CAD build for the part. Positions are in the model's coordinates, mm. Face numbers are marked on the shaded views. A direction names the side the tool comes from. Coordinates: 2 decimals unless noted, no trailing zeros. Loops run counter-clockwise (first coordinate to the right, second up) from the corner with the lowest first, then second, coordinate; pieces in that order, holes last. Notation, with made-up numbers: (86.25, 16) -> (118.25, 16) arc R21 ccw to (118.25, 29) -> close; hole circle Ø2 at (59, 41). An arc over 180 degrees is marked (long way). Write each question's results on one line, items separated by ' | '.
from build123d import *

# Parameters (mm, degrees)
SKETCH1_W           = 8
SKETCH1_H           = 40
BOSS_EXTRUDE1_DEPTH = 5
SKETCH3_W           = 8
SKETCH3_H           = 8
BOSS_EXTRUDE3_DEPTH = 70
SKETCH4_R           = 4
BOSS_EXTRUDE4_DEPTH = 30
SKETCH5_R           = 0.773565548
SKETCH5_R_2         = 0.768304054
SKETCH5_R_3         = 0.726526648
SKETCH5_R_4         = 0.707209462
SKETCH5_R_5         = 0.715862797
SKETCH5_R_6         = 0.812614346
CUT_EXTRUDE1_DEPTH  = 10
FILLET1_R           = 3


with BuildPart() as part:
    # Sketch1 → Boss-Extrude1 (new body)
    with BuildSketch(Plane.XY):
        with Locations((4, 20)):
            Rectangle(SKETCH1_W, SKETCH1_H)
    extrude(amount=BOSS_EXTRUDE1_DEPTH)

    # Sketch3 → Boss-Extrude3 (add)
    with BuildSketch(Plane.XY.offset(5)):
        with Locations((4, 20)):
            Rectangle(SKETCH3_W, SKETCH3_H)
    extrude(amount=BOSS_EXTRUDE3_DEPTH)

    # Sketch4 → Boss-Extrude4 (add)
    with BuildSketch(Plane.XY.offset(75)):
        with Locations((4, 20)):
            Circle(SKETCH4_R)
    extrude(amount=BOSS_EXTRUDE4_DEPTH)

    # Sketch5 → Cut-Extrude1 (cut)
    with BuildSketch(Plane.XY.offset(5)):
        with Locations((4, 3.47)):
            Circle(SKETCH5_R)
        with Locations((4, 6.47)):
            Circle(SKETCH5_R_2)
        with Locations((4, 9.47)):
            Circle(SKETCH5_R_3)
        with Locations((4, 30.53)):
            Circle(SKETCH5_R_4)
        with Locations((4, 33.53)):
            Circle(SKETCH5_R_5)
        with Locations((4, 36.53)):
            Circle(SKETCH5_R_6)
    extrude(amount=-CUT_EXTRUDE1_DEPTH, mode=Mode.SUBTRACT)

    # Fillet1
    fillet1_edges = [part.edges().sort_by_distance(p)[0] for p in [
        (4, 16, 5),
        (4, 24, 5),
    ]]
    fillet(fillet1_edges, radius=FILLET1_R)


solid = part.part
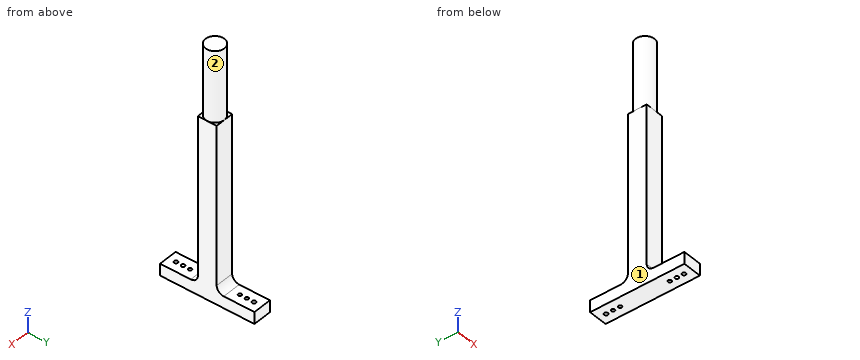
1) Pin check, flat tips, straight feed: pin 1 (1.5 mm diameter, centred on x = 1.5, y = 35.5, fed in from -Z); pin 2 (1 mm diameter, centred on x = 2, z = 92.5, fed in from +Y); pin 3 (0.9 mm diameter, centred on x = 4, y = 33.53, fed in from +Z); pin 4 (1.8 mm diameter, centred on x = 4, y = 30.53, fed in from +Z). Stop position of each tip, or through.
Outcome:
pin 1: stops at z = 0 | pin 2: stops at y = 23.71 | pin 3: passes through | pin 4: stops at z = 5
2) Slice it at C-C (y = 22). Write the cut outline in (x, z), then the cut area to 3 significant figures.
Outcome:
outline: (0, 0) -> (8, 0) -> (8, 75) -> (7.46, 75) -> (7.46, 105) -> (0.54, 105) -> (0.54, 75) -> (0, 75) -> close | area: 808 mm^2
3) Which spindle directions (+Z, -Z, +X, -X, +Y, -Y) get a long thin tool onto all of the face, cutting with end or side? Do the marked faces 1 and 2. Say none if no direction does.
Outcome:
face 1: +Z, -Z, -X, +Y, -Y | face 2: +Z
4) Slice it at D-D (z = 63). Write the cut outline in (x, y).
Outcome:
outline: (0, 16) -> (8, 16) -> (8, 24) -> (0, 24) -> close
5) Slice it at A-A (x = 5.75). Write the cut outline in (y, z), then the cut area to 3 significant figures.
Outcome:
outline: (0, 0) -> (40, 0) -> (40, 5) -> (27, 5) arc R3 cw to (24, 8) -> (24, 75) -> (23.6, 75) -> (23.6, 105) -> (16.4, 105) -> (16.4, 75) -> (16, 75) -> (16, 8) arc R3 cw to (13, 5) -> (0, 5) -> close | area: 980 mm^2
6) Drill centre lines: L1, parallel to X at y = 36.53, z = 1.45; L2, parallel to Y at x = 2.5, z = 53; L3, parallel to Z at x = 7.5, y = 2.5. Where is each one in solid material? Low to high. Write a range as from..to.
Outcome:
L1: x = 0..3.19, 4.81..8 | L2: y = 16..24 | L3: z = 0..5
7) Slice it at B-B (z = 93.5). Write the cut outline in (x, y), then the cut area to 3 significant figures.
Outcome:
outline: circle Ø8 at (4, 20) | area: 50.3 mm^2
